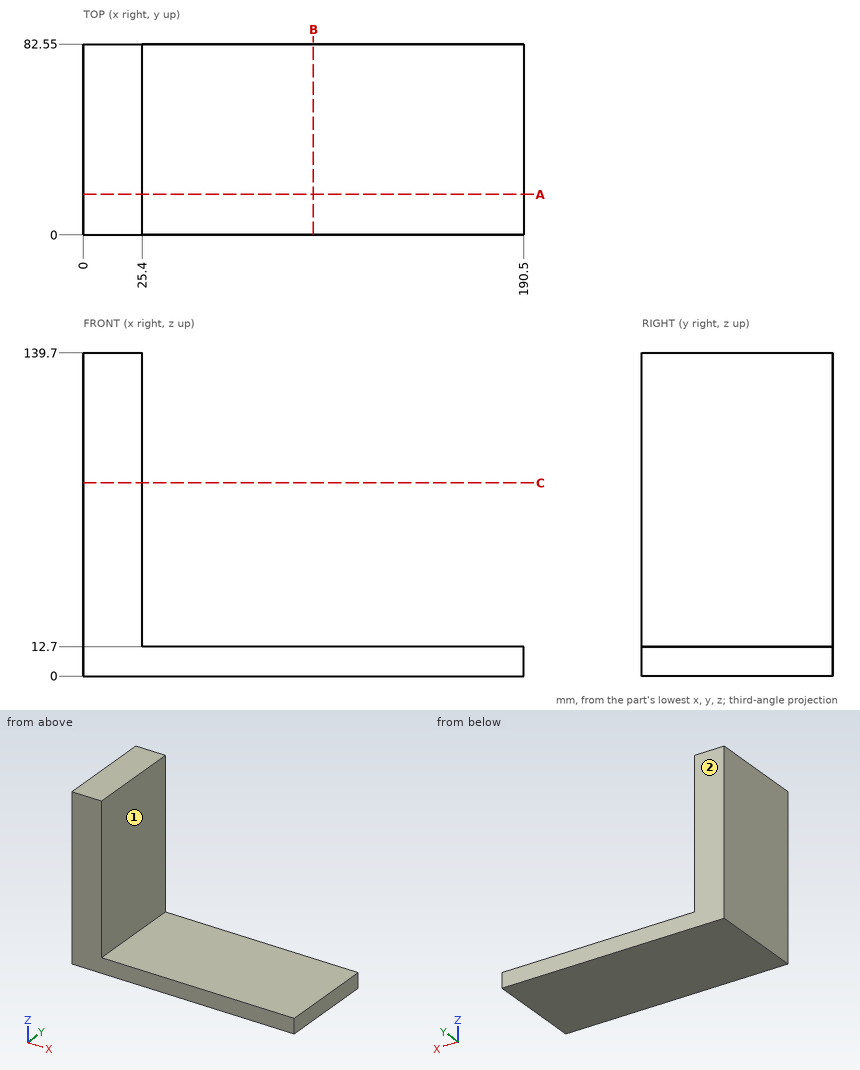
For this review, use the dimensioned drawing (mm, ordinates from the lowest corner) and the shaded views. A direction names the side the tool comes from. Give positions to 0.01 mm unless a question says otherwise; leave off trailing zeros. Write each loop counter-clockwise with the first axis right and the second up, starting at its lowest first coordinate (ties: lowest second). Pieces come first, ordered by that corner, then holes. Notation, with made-up numbers: M 30.25,-16.5 L 44.25,-16.5 A33 ccw 44.25,15.5 Z; hole C -25,34.25 d1. An arc over 180 degrees is marked long. Write item = value, one per line. Start each with the question number.
Q1. Clearance check with flat-ended pins moving along their axes: pin 1 (10 mm diameter, centred on y = 56, z = 53, fed in from +X); pin 2 (25 mm diameter, centred on x = 77, y = 34.5, fed in from +Z). State where each tip first meets the part, or that it passes through.
Q2. Machinability: for the marked faces 1 and 2, which of the approach directions +Z, -Z, +X, -X, +Y, -Y give a long, thin tool a straight path to every point of the face, cutting with its end or side? Answer none if there is none.
Q3. For line 1 (Z direction, x = 141.5, y = 73.5); line 2 (X direction, y = 74.5, z = 92), list the stretches that pass through material, from the lowest coordinate up.
Q4. We need section A-A (y = 17.5). State the section outline as (x, z) points, plus the area to 3 significant figures.
Q5. We need section C-C (z = 83.5). State the section outline as (x, y) points.
Q6. We need section B-B (x = 99.5). State the section outline as (y, z) points.
Result set:
q1.pin_1 = 25.4
q1.pin_2 = 12.7
q2.face_1 = +Z, +X, +Y, -Y
q2.face_2 = +Z, -Z, +X, -X, +Y
q3.line_1 = 0 to 12.7
q3.line_2 = 0 to 25.4
q4.outline = M 0,0 L 190.5,0 L 190.5,12.7 L 25.4,12.7 L 25.4,139.7 L 0,139.7 Z
q4.area = 5,650 mm2
q5.outline = M 0,0 L 25.4,0 L 25.4,82.55 L 0,82.55 Z
q6.outline = M 0,0 L 82.55,0 L 82.55,12.7 L 0,12.7 Z
